```python
from build123d import *

# Parameters (mm, degrees)
FILLET1_R = 2.54


with BuildPart() as part:
    # Sketch2 → Revolve1 (revolve)
    with BuildSketch(Plane.XY):
        Polygon((4.445, 0), (11.1125, 0), (11.1125, 13.589), (7.9375, 16.764), (11.1125, 19.939), (11.1125, 33.528), (4.445, 33.528), align=None)
    revolve(axis=Axis((0, 0, 0), (0, 1, 0)))

    # Fillet1
    fillet1_edges = [part.edges().sort_by_distance(p)[0] for p in [
        (-7.9375, 16.764, 0),
    ]]
    fillet(fillet1_edges, radius=FILLET1_R)


solid = part.part
```
Read the model definition and answer for the solid it produces. Units are mm, in the model's axes. Coordinates: 2 decimals unless noted, no trailing zeros. Write each loop counter-clockwise with the first axis right and the second up, starting at its lowest first coordinate (ties: lowest second). Pieces come first, ordered by that corner, then holes. Notation, with made-up numbers: (32, 57) - (58, 57) arc R30 cw to (58, 94) - close; hole circle Ø5 at (58, -18.75). An arc over 180 degrees is marked (long way). Answer as a JSON object with one key per item and string values. Group by question number.
1. Each of these flat-tipped pins is pushed along its axis until it touches: P1, Ø1, axis at y = 10, z = -4.5, coming from the +X side; P2, Ø6, axis at y = 30, z = 3.5, coming from the -X side; P3, Ø4, axis at x = 8.5, y = 24, coming from the +Z side. Where does it stop, or does it pass through?
2. A cutting plane is placed at A-A (y = 9). Determine the outline of the cut face in (x, z) (1 decimal), plus the area to 3 significant figures.
3. Consider L1, parallel to Z at x = 0, y = 25 (1 decimal); L2, parallel to X at y = 12.5, z = -2. Determine where each line is inside the solid, lowest interval first. Write a range as [from, to].
4. A cutting plane is placed at B-B (y = 19.5). Determine the outline of the cut face in (x, z) (1 decimal).
5. The mould has two halves that part along Z. Classify faces 1 (the cylindrical face through (-0.96, 16.53, 4.34)), 2 (the flat face through (0, 33.528, 5)), 3 (the cylindrical face through (10.6, 26.83, -3.34)): +Z half, -Z half, draft (parallel to the pull), parting line (faces both ways), or undercut.
Worked out:
{
 "1": {"P1": "stops at x = 10.37", "P2": "stops at x = -11.1", "P3": "stops at z = 9.01"},
 "2": {"outline": "circle Ø22.2 at (0, 0); hole circle Ø8.9 at (0, 0)", "area": "326 mm²"},
 "3": {"L1": "z = [-11.1, -4.4], [4.4, 11.1]", "L2": "x = [-10.93, -3.97], [3.97, 10.93]"},
 "4": {"outline": "circle Ø21.3 at (0, 0); hole circle Ø8.9 at (0, 0)"},
 "5": {"face 1": "undercut", "face 2": "draft", "face 3": "parting line"}
}
